Input: part model. Units: mm. Frame: model coordinates. Round coordinates to 2 decimals unless told otherwise and drop trailing zeros. Loops run counter-clockwise (first coordinate to the right, second up) from the corner with the lowest first, then second, coordinate; pieces in that order, holes last.
1) Section D-D, the plane x = 4.25. Return loops of the section in (y, z).
2) Ray query, line 1 along Y through (x, z) = (0, 3.15); line 2 along Y through (x, z) = (1.25, 5.5); line 3 along X through (y, z) = (-1, 1.4). Return the intervals inside material, ascending.
3) Draft query along Y for faces 1 (the face through (4.2, 0.1, 0)), 2 (the face through (0, 5.629, 3)), 3 (the face through (-0.867, -3.905, 2.958)), 4 (the face through (-4.898, -2.775, 2.958)). Return one class per face: pulls with the +Y half, pulls with the -Y half, needs draft (parallel to the pull), parting line crosses it, or undercut.
4) Section C-C, the plane y = 1.25. Return loops of the section in (x, z).
5) Section A-A, the plane x = 0. Return loops of the section in (y, z), and give its area (4 significant figures).
6) Section B-B, the plane z = 2.75. Return loops of the section in (x, y), and give its area (3 significant figures).
7) First-contact query: pin 1 (6 mm diameter, centred on x = 1, y = -3.5, fed in from +Z); pin 2 (2 mm diameter, centred on x = -4.5, z = 3, fed in from +Y); pin 3 (2 mm diameter, centred on y = -1.5, z = 4.5, fed in from -X). Flat tips, straight axial feed; report the tip coordinate or a pass-through.
from build123d import *

# Parameters (mm, degrees)
BOSS_EXTRUDE1_DEPTH = 6
SKETCH2_R           = 4
CUT_EXTRUDE1_DEPTH  = 6


with BuildPart() as part:
    # Sketch1 → Boss-Extrude1 (new body)
    with BuildSketch(Plane.XY):
        Polygon((6.5, 0), (3.25, 5.629165125), (-3.25, 5.629165125), (-6.5, 0), (-3.25, -5.629165125), (3.25, -5.629165125), align=None)
    extrude(amount=BOSS_EXTRUDE1_DEPTH)

    # Sketch2 → Cut-Extrude1 (cut)
    with BuildSketch(Plane.XY):
        Circle(SKETCH2_R)
    extrude(amount=CUT_EXTRUDE1_DEPTH, mode=Mode.SUBTRACT)


solid = part.part
Final values:
1. outline: (-3.9, 0) - (3.9, 0) - (3.9, 6) - (-3.9, 6) - close
2. line 1: y = -5.63 to -4, 4 to 5.63
2. line 2: y = -5.63 to -3.8, 3.8 to 5.63
2. line 3: x = -5.92 to -3.87, 3.87 to 5.92
3. face 1: needs draft
3. face 2: pulls with the +Y half
3. face 3: undercut
3. face 4: pulls with the -Y half
4. outline: (-5.78, 0) - (-3.8, 0) - (-3.8, 6) - (-5.78, 6) - close; (3.8, 0) - (5.78, 0) - (5.78, 6) - (3.8, 6) - close
5. outline: (-5.63, 0) - (-4, 0) - (-4, 6) - (-5.63, 6) - close; (4, 0) - (5.63, 0) - (5.63, 6) - (4, 6) - close
5. area: 19.55 mm2
6. outline: (-6.5, 0) - (-3.25, -5.63) - (3.25, -5.63) - (6.5, 0) - (3.25, 5.63) - (-3.25, 5.63) - close; hole circle Ø8 at (0, 0)
6. area: 59.5 mm2
7. pin 1: stops at z = 6
7. pin 2: stops at y = 5.2
7. pin 3: stops at x = -6.21
